from build123d import *

# Parameters (mm, degrees)
BOSS_EXTRUDE1_DEPTH = 3.175
BOSS_EXTRUDE2_DEPTH = 3.175
SKETCH3_R           = 19.05
SKETCH3_R_2         = 15.875
BOSS_EXTRUDE3_DEPTH = 6.35
SKETCH4_R           = 2.54
CUT_EXTRUDE1_DEPTH  = 34.89972345
CHAMFER1_SIZE       = 1.27


with BuildPart() as part:
    # Sketch1 → Boss-Extrude1 (new body)
    with BuildSketch(Plane(origin=(0, 0, 0), x_dir=(1, 0, 0), z_dir=(0, 1, 0))):
        with BuildLine():
            Line((-15.875, -22.225), (15.875, -22.225))
            ThreePointArc((15.875, -22.225), (20.365128061, -20.365128061), (22.225, -15.875))
            Line((22.225, -15.875), (22.225, 15.875))
            ThreePointArc((22.225, 15.875), (20.365128061, 20.365128061), (15.875, 22.225))
            Line((15.875, 22.225), (-15.875, 22.225))
            ThreePointArc((-15.875, 22.225), (-20.365128061, 20.365128061), (-22.225, 15.875))
            Line((-22.225, 15.875), (-22.225, -15.875))
            ThreePointArc((-22.225, -15.875), (-20.365128061, -20.365128061), (-15.875, -22.225))
        make_face()
    extrude(amount=BOSS_EXTRUDE1_DEPTH)

    # Sketch2 → Boss-Extrude2 (add)
    with BuildSketch(Plane(origin=(0, 3.175, 0), x_dir=(1, 0, 0), z_dir=(0, 1, 0))):
        with BuildLine():
            Line((9.779188038, 17.653644576), (-8.104452463, 17.653644576))
            ThreePointArc((-8.104452463, 17.653644576), (-9.392376749, 18.004386475), (-10.324608902, 18.959746126))
            ThreePointArc((-10.324608902, 18.959746126), (-12.655189283, 21.348145252), (-15.875, 22.225))
            ThreePointArc((-15.875, 22.225), (-20.365128061, 20.365128061), (-22.225, 15.875))
            ThreePointArc((-22.225, 15.875), (-21.348011707, 12.654962289), (-18.959285714, 10.324353044))
            ThreePointArc((-18.959285714, 10.324353044), (-18.003795317, 9.392109345), (-17.653, 8.104094261))
            Line((-17.653, 8.104094261), (-17.653, -8.104094261))
            ThreePointArc((-17.653, -8.104094261), (-18.003795317, -9.392109345), (-18.959285714, -10.324353044))
            ThreePointArc((-18.959285714, -10.324353044), (-21.348011707, -12.654962289), (-22.225, -15.875))
            ThreePointArc((-22.225, -15.875), (-20.365128061, -20.365128061), (-15.875, -22.225))
            ThreePointArc((-15.875, -22.225), (-12.655189283, -21.348145252), (-10.324608902, -18.959746126))
            ThreePointArc((-10.324608902, -18.959746126), (-9.392376749, -18.004386475), (-8.104452463, -17.653644576))
            Line((-8.104452463, -17.653644576), (8.104452463, -17.653644576))
            ThreePointArc((8.104452463, -17.653644576), (9.392376749, -18.004386475), (10.324608902, -18.959746126))
            ThreePointArc((10.324608902, -18.959746126), (12.655189283, -21.348145252), (15.875, -22.225))
            ThreePointArc((15.875, -22.225), (20.365128061, -20.365128061), (22.225, -15.875))
            ThreePointArc((22.225, -15.875), (21.348011707, -12.654962289), (18.959285714, -10.324353044))
            ThreePointArc((18.959285714, -10.324353044), (18.003795317, -9.392109345), (17.653, -8.104094261))
            Line((17.653, -8.104094261), (17.653, 8.104094261))
            ThreePointArc((17.653, 8.104094261), (18.003795317, 9.392109345), (18.959285714, 10.324353044))
            ThreePointArc((18.959285714, 10.324353044), (21.348011707, 12.654962289), (22.225, 15.875))
            ThreePointArc((22.225, 15.875), (20.365128061, 20.365128061), (15.875, 22.225))
            ThreePointArc((15.875, 22.225), (12.065268583, 20.955201426), (9.779188038, 17.653644576))
        make_face()
    extrude(amount=BOSS_EXTRUDE2_DEPTH)

    # Sketch3 → Boss-Extrude3 (add)
    with BuildSketch(Plane.XZ):
        with Locations(Location((0, 0, 0), (0, 0, 90))):
            Circle(SKETCH3_R)
        with Locations(Location((0, 0, 0), (0, 0, 270))):
            Circle(SKETCH3_R_2, mode=Mode.SUBTRACT)
    extrude(amount=BOSS_EXTRUDE3_DEPTH)

    # Sketch4 → Cut-Extrude1 (cut, through all)
    with BuildSketch(Plane(origin=(0, 6.35, 0), x_dir=(1, 0, 0), z_dir=(0, 1, 0))):
        with Locations(Location((-15.875, 15.875, 0), (0, 0, 270))):
            Circle(SKETCH4_R)
        with Locations(Location((15.875, 15.875, 0), (0, 0, 270))):
            Circle(SKETCH4_R)
        with Locations(Location((-15.875, -15.875, 0), (0, 0, 270))):
            Circle(SKETCH4_R)
        with Locations(Location((15.875, -15.875, 0), (0, 0, 270))):
            Circle(SKETCH4_R)
    extrude(amount=-CUT_EXTRUDE1_DEPTH, mode=Mode.SUBTRACT)

    # Chamfer1
    chamfer1_edges = [part.edges().sort_by_distance(p)[0] for p in [
        (-20.365314283, 6.35, -20.36494183),
        (-20.365314283, 6.35, 20.36494183),
        (-9.392376749, 6.35, -18.004386475),
        (19.836937806, 6.35, -20.837413609),
        (0.837367788, 6.35, -17.653644576),
        (18.003795317, 6.35, -9.392109345),
        (17.653, 6.35, 0),
        (18.003795317, 6.35, 9.392109345),
        (-18.003795317, 6.35, -9.392109345),
        (20.365314283, 6.35, 20.36494183),
        (-17.653, 6.35, 0),
        (9.392376749, 6.35, 18.004386475),
        (-18.003795317, 6.35, 9.392109345),
        (0, 6.35, 17.653644576),
        (-9.392376749, 6.35, 18.004386475),
    ]]
    chamfer(chamfer1_edges, length=CHAMFER1_SIZE)
    chamfer1_2_edges = [part.edges().sort_by_distance(p)[0] for p in [
        (0, -6.35, -19.05),
    ]]
    chamfer(chamfer1_2_edges, length=CHAMFER1_SIZE)
    chamfer1_3_edges = [part.edges().sort_by_distance(p)[0] for p in [
        (0, -6.35, 15.875),
    ]]
    chamfer(chamfer1_3_edges, length=CHAMFER1_SIZE)
    # the kernel refuses this chamfer: 1.27 mm, written as the material it takes off along each edge
    with BuildSketch(Plane(origin=(-22.225, 3.175, -19.141037395), x_dir=(-0.02749587661058728, -0.9996219169112966, 0), z_dir=(0, 0, 1))) as chamfer1_4_piece_1_section:
        with BuildLine():
            Line((1.306414958, 0), (-0.071814887, 1.304439598))
            Line((-0.071814887, 1.304439598), (-0.097205283, 1.303741203))
            ThreePointArc((-0.097205283, 1.303741203), (-0.043344118, 0.652015244), (-0.025390397, -0.000698395))
            Line((-0.025390397, -0.000698395), (0.000698395, -0.025390397))
            ThreePointArc((0.000698395, -0.025390397), (0.653412034, -0.007436675), (1.307113353, -0.025390397))
            Line((1.307113353, -0.025390397), (1.306414958, 0))
        make_face()
    chamfer1_4_piece_1 = extrude(amount=38.282074789, mode=Mode.PRIVATE)
    chamfer1_4_piece_1 = chamfer1_4_piece_1 - Plane(origin=(-15.875, 2.735416382, -15.875), x_dir=(0, 0, -1), z_dir=(0, -1, 0)) * Cylinder(6.35, 82, mode=Mode.PRIVATE)
    chamfer1_4_piece_1 = chamfer1_4_piece_1 - Plane(origin=(-15.875, 2.735416382, 15.875), x_dir=(-1, 0, 0), z_dir=(0, -1, 0)) * Cylinder(6.35, 82, mode=Mode.PRIVATE)
    add(chamfer1_4_piece_1, mode=Mode.SUBTRACT)
    # the kernel refuses this chamfer: 1.27 mm, written as the material it takes off along each edge
    with BuildSketch(Plane(origin=(19.141037395, 3.175, -22.225), x_dir=(0, -0.9996219169112966, -0.02749587661058728), z_dir=(-1, 0, 0))) as chamfer1_5_piece_1_section:
        with BuildLine():
            Line((1.306414958, 0), (-0.071814887, 1.304439598))
            Line((-0.071814887, 1.304439598), (-0.097205283, 1.303741203))
            ThreePointArc((-0.097205283, 1.303741203), (-0.043344118, 0.652015244), (-0.025390397, -0.000698395))
            Line((-0.025390397, -0.000698395), (0.000698395, -0.025390397))
            ThreePointArc((0.000698395, -0.025390397), (0.653412034, -0.007436675), (1.307113353, -0.025390397))
            Line((1.307113353, -0.025390397), (1.306414958, 0))
        make_face()
    chamfer1_5_piece_1 = extrude(amount=38.282074789, mode=Mode.PRIVATE)
    chamfer1_5_piece_1 = chamfer1_5_piece_1 - Plane(origin=(-15.875, 2.735416382, -15.875), x_dir=(0, 0, -1), z_dir=(0, -1, 0)) * Cylinder(6.35, 82, mode=Mode.PRIVATE)
    chamfer1_5_piece_1 = chamfer1_5_piece_1 - Plane(origin=(15.875, 2.735416382, -15.875), x_dir=(1, 0, 0), z_dir=(0, -1, 0)) * Cylinder(6.35, 82, mode=Mode.PRIVATE)
    add(chamfer1_5_piece_1, mode=Mode.SUBTRACT)
    # the kernel refuses this chamfer: 1.27 mm, written as the material it takes off along each edge
    with BuildSketch(Plane(origin=(-19.141037395, 3.175, 22.225), x_dir=(0, -0.9996219169112966, 0.02749587661058728), z_dir=(1, 0, 0))) as chamfer1_6_piece_1_section:
        with BuildLine():
            Line((1.306414958, 0), (-0.071814887, 1.304439598))
            Line((-0.071814887, 1.304439598), (-0.097205283, 1.303741203))
            ThreePointArc((-0.097205283, 1.303741203), (-0.043344118, 0.652015244), (-0.025390397, -0.000698395))
            Line((-0.025390397, -0.000698395), (0.000698395, -0.025390397))
            ThreePointArc((0.000698395, -0.025390397), (0.653412034, -0.007436675), (1.307113353, -0.025390397))
            Line((1.307113353, -0.025390397), (1.306414958, 0))
        make_face()
    chamfer1_6_piece_1 = extrude(amount=38.282074789, mode=Mode.PRIVATE)
    chamfer1_6_piece_1 = chamfer1_6_piece_1 - Plane(origin=(-15.875, 2.735416383, 15.875), x_dir=(-1, 0, 0), z_dir=(0, -1, 0)) * Cylinder(6.35, 82, mode=Mode.PRIVATE)
    chamfer1_6_piece_1 = chamfer1_6_piece_1 - Plane(origin=(15.875, 2.735416383, 15.875), x_dir=(0, 0, 1), z_dir=(0, -1, 0)) * Cylinder(6.35, 82, mode=Mode.PRIVATE)
    add(chamfer1_6_piece_1, mode=Mode.SUBTRACT)
    # the kernel refuses this chamfer: 1.27 mm, written as the material it takes off along each edge
    with BuildSketch(Plane(origin=(22.225, 3.175, 19.141037395), x_dir=(0.02749587661058728, -0.9996219169112966, 0), z_dir=(0, 0, -1))) as chamfer1_7_piece_1_section:
        with BuildLine():
            Line((1.306414958, 0), (-0.071814887, 1.304439598))
            Line((-0.071814887, 1.304439598), (-0.097205283, 1.303741203))
            ThreePointArc((-0.097205283, 1.303741203), (-0.043344118, 0.652015244), (-0.025390397, -0.000698395))
            Line((-0.025390397, -0.000698395), (0.000698395, -0.025390397))
            ThreePointArc((0.000698395, -0.025390397), (0.653412034, -0.007436675), (1.307113353, -0.025390397))
            Line((1.307113353, -0.025390397), (1.306414958, 0))
        make_face()
    chamfer1_7_piece_1 = extrude(amount=38.282074789, mode=Mode.PRIVATE)
    chamfer1_7_piece_1 = chamfer1_7_piece_1 - Plane(origin=(15.875, 2.735416383, -15.875), x_dir=(1, 0, 0), z_dir=(0, -1, 0)) * Cylinder(6.35, 82, mode=Mode.PRIVATE)
    chamfer1_7_piece_1 = chamfer1_7_piece_1 - Plane(origin=(15.875, 2.735416383, 15.875), x_dir=(0, 0, 1), z_dir=(0, -1, 0)) * Cylinder(6.35, 82, mode=Mode.PRIVATE)
    add(chamfer1_7_piece_1, mode=Mode.SUBTRACT)


solid = part.part
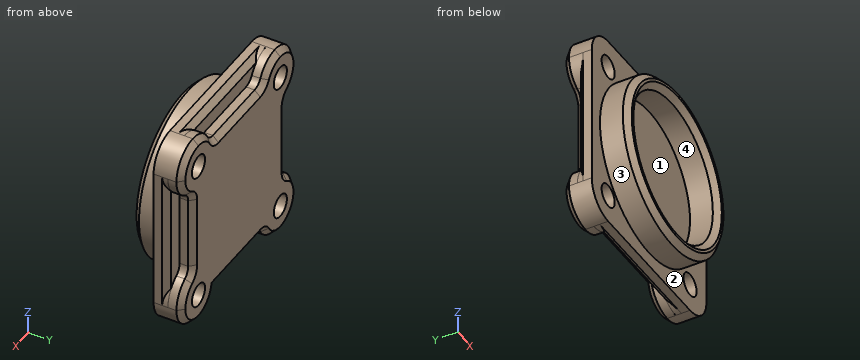
For this review, take the finished solid that the model builds, in its own axes (mm). Face numbers are marked on the shaded views. Round coordinates to 2 decimals unless told otherwise and drop trailing zeros. Write each loop counter-clockwise with the first axis right and the second up, starting at its lowest first coordinate (ties: lowest second). Pieces come first, ordered by that corner, then holes. Notation, with made-up numbers: (12, 67.25) -> (63, 67.25) arc R24 cw to (63, 91.25) -> close; hole circle Ø7 at (-26, 11.5). An arc over 180 degrees is marked (long way). Use CSV: the item, a comma, the result in double quotes.
(1) Consider section A-A, the plane y = 1. Give the boundary of the cut face in (x, z) (3 decimals), plus the area to 3 significant figures.
Computed values:
outline,"(-22.225, -15.875) arc R6.35 ccw to (-15.875, -22.225) -> (15.875, -22.225) arc R6.35 ccw to (22.225, -15.875) -> (22.225, 15.875) arc R6.35 ccw to (15.875, 22.225) -> (-15.875, 22.225) arc R6.35 ccw to (-22.225, 15.875) -> close; hole circle Ø5.08 at (-15.875, -15.875); hole circle Ø5.08 at (-15.875, 15.875); hole circle Ø5.08 at (15.875, -15.875); hole circle Ø5.08 at (15.875, 15.875)"
area,"1,860 mm²"
(2) Consider section C-C, the plane z = 0. Give the boundary of the cut face in (x, y) (3 decimals), plus the area to 3 significant figures.
Computed values:
outline,"(-22.225, 0) -> (-19.05, 0) -> (-19.05, -5.08) -> (-17.78, -6.35) -> (-17.145, -6.35) -> (-15.875, -5.08) -> (-15.875, 0) -> (15.875, 0) -> (15.875, -5.08) -> (17.145, -6.35) -> (17.78, -6.35) -> (19.05, -5.08) -> (19.05, 0) -> (22.225, 0) -> (22.225, 1.905) -> (20.955, 3.175) -> (17.653, 3.175) -> (17.653, 5.08) -> (16.383, 6.35) -> (-16.383, 6.35) -> (-17.653, 5.08) -> (-17.653, 3.175) -> (-20.955, 3.175) -> (-22.225, 1.905) -> close"
area,"287 mm²"
(3) Draft analysis for pull direction Z (two halves, no side actions). For the marked faces 1, 2, 3 and 4, state which applies: +Z half, -Z half, draft (parallel to the pull), parting line (faces both ways), or undercut.
Computed values:
face 1,"undercut"
face 2,"draft"
face 3,"parting line"
face 4,"undercut"
(4) To check wall thickness, follow L1, parallel to X at y = 4.25, z = 14; L2, parallel to X at y = -0.5, z = -0.5; L3, parallel to Z at x = 0.5, y = 4.5. State the ranges of each line that lie inside material, in increasing order. Write a range as [from, to].
Computed values:
L1,"[-21.94, -17.59], [-14.16, 14.16], [17.59, 21.94]"
L2,"[-19.04, -15.87], [15.87, 19.04]"
L3,"[-17.65, 17.65]"
(5) Clearance check with flat-ended pins moving along their axes: P1, Ø2, axis at y = 4.5, z = -17.5, coming from the -X side; P2, Ø12, axis at x = -3.5, z = -6.5, coming from the -Y side; P3, Ø2, axis at y = -1.5, z = -12.5, coming from the +X side; P4, Ø4, axis at x = -15.875, z = -15.875, coming from the +Y side. State where each tip first meets the part, or that it passes through.
Computed values:
P1,"x = -22.19"
P2,"y = 0"
P3,"x = 15.19"
P4,"through"
(6) Consider section B-B, the plane x = 0. Give the boundary of the cut face in (y, z) (3 decimals).
Computed values:
outline,"(-6.35, -17.78) -> (-5.08, -19.05) -> (0, -19.05) -> (0, -22.225) -> (1.905, -22.225) -> (3.175, -20.955) -> (3.175, -17.654) -> (5.08, -17.654) -> (6.35, -16.384) -> (6.35, 16.384) -> (5.08, 17.654) -> (3.175, 17.654) -> (3.175, 20.955) -> (1.905, 22.225) -> (0, 22.225) -> (0, 19.05) -> (-5.08, 19.05) -> (-6.35, 17.78) -> (-6.35, 17.145) -> (-5.08, 15.875) -> (0, 15.875) -> (0, -15.875) -> (-5.08, -15.875) -> (-6.35, -17.145) -> close"
(7) Consider section D-D, the plane y = -2.25. Give the boundary of the cut face in (x, z) (3 decimals).
Computed values:
outline,"circle Ø38.1 at (0, 0); hole circle Ø31.75 at (0, 0)"
